Could you check a few things on this drawing? It's one solid part, dimensions in mm from its lowest x, y, z. A direction names the side the tool comes from. Give positions to 0.01 mm unless a question says otherwise; leave off trailing zeros. Order: outer loops, then holes, each group sorted by start corner. A loop starts at its lowest first (then second) coordinate and runs counter-clockwise, first axis right, second up. Notation, with made-up numbers: (56.25, 18) - (75.25, 18) arc R29 cw to (75.25, 38) - close; hole circle Ø11 at (28.25, -39). An arc over 180 degrees is marked (long way). Put each result on its own line as item: value.
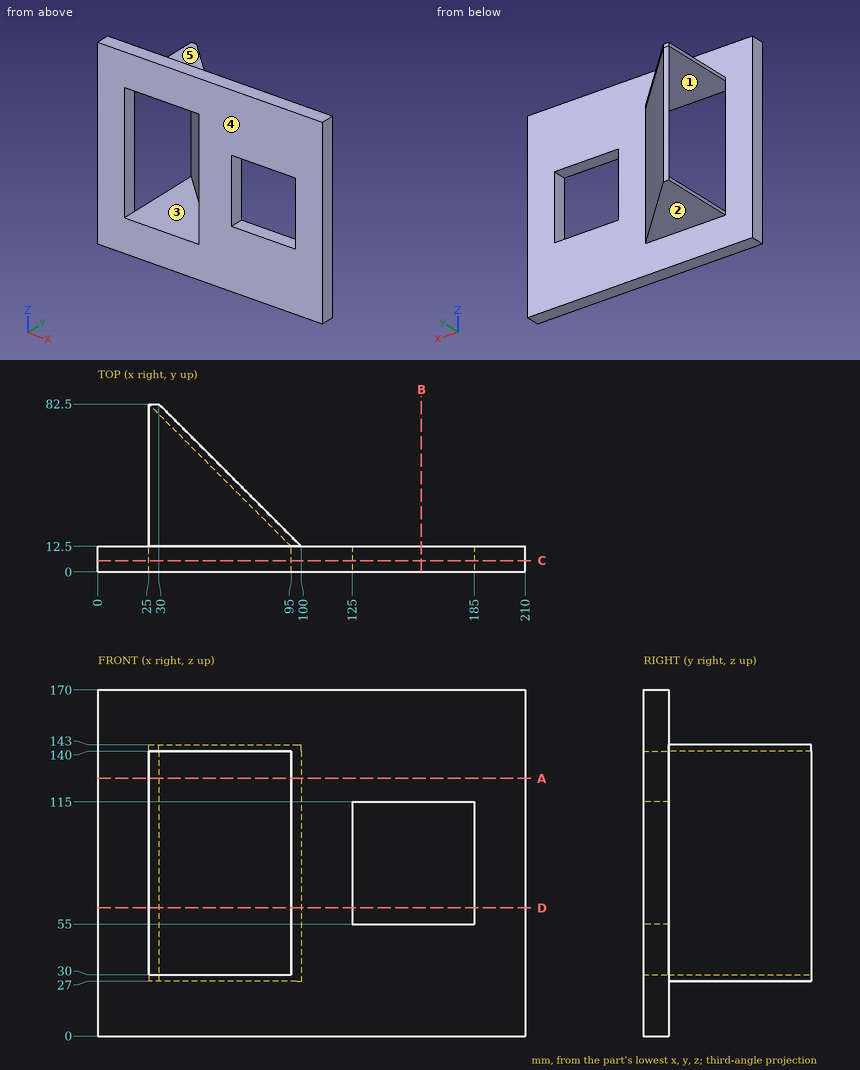
1) Which directions (+Z, -Z, +X, -X, +Y, -Y) give clear straight access to the entire face, cutting with the end or side of a thin tool? Please do the marked faces 4 and 5.
Filled in:
face 4: +Z, -Z, +X, -X, -Y
face 5: +Z, +X, -X, +Y
2) Suppose I cut it at D-D, the plane z = 63. List the corners of the cut face in (x, y) for me.
Filled in:
outline: (0, 0) - (25, 0) - (25, 12.5) - (0, 12.5) - close; (25, 82.5) - (95, 12.5) - (95, 0) - (125, 0) - (125, 12.5) - (100, 12.5) - (30, 82.5) - close; (185, 0) - (210, 0) - (210, 12.5) - (185, 12.5) - close
3) Suppose I cut it at A-A, the plane z = 126.5. List the corners of the cut face in (x, y) for me.
Filled in:
outline: (0, 0) - (25, 0) - (25, 12.5) - (0, 12.5) - close; (25, 82.5) - (95, 12.5) - (95, 0) - (210, 0) - (210, 12.5) - (100, 12.5) - (30, 82.5) - close
4) Suppose I cut it at B-B, the plane x = 159. List the corners of the cut face in (y, z) for me.
Filled in:
outline: (0, 0) - (12.5, 0) - (12.5, 55) - (0, 55) - close; (0, 115) - (12.5, 115) - (12.5, 170) - (0, 170) - close
5) We'd pull the mould along X, two halves only. Please class the marked faces 1, 2 and 3: pulls with the +X half, pulls with the -X half, needs draft (parallel to the pull), parting line crosses it, or undercut.
Filled in:
face 1: undercut
face 2: needs draft
face 3: undercut
6) Suppose I cut it at C-C, the plane y = 5.5. List the corners of the cut face in (x, z) for me, and give its area (3 significant figures).
Filled in:
outline: (0, 0) - (210, 0) - (210, 170) - (0, 170) - close; hole (25, 30) - (95, 30) - (95, 140) - (25, 140) - close; hole (125, 55) - (185, 55) - (185, 115) - (125, 115) - close
area: 24,400 mm^2
7) If I drill on line 1 (X direction, y = 9, z = 93.5); line 2 (Z direction, x = 68, y = 17.5); line 3 (Z direction, x = 138, y = 10), over which ranges is the centre line in solid material (lowest first)? Write a range as [from, to].
Filled in:
line 1: x = [0, 25], [95, 125], [185, 210]
line 2: z = [27, 30], [140, 143]
line 3: z = [0, 55], [115, 170]
8) I'm going to push flat-ended pins straight in: pin 1 (3 mm diameter, centred on y = 58.5, z = 137, fed in from -X); pin 2 (21 mm diameter, centred on x = 51, y = 48.5, fed in from -Z); pin 3 (0.9 mm diameter, centred on y = 60.5, z = 141.5, fed in from -X). Where does each tip first touch, or does it pass through?
Filled in:
pin 1: stops at x = 47.5
pin 2: stops at z = 27
pin 3: stops at x = 25
